Autodesk Fusion 360 part; units mm, degrees
sketch "Obturator" plane through (0, 0, 0) normal (1, 0, 0) x (0, 1, 0)
  circle A0 centre (0, 0) radius 80
  line L0 (85, 85) -> (-85, 85)
  line L1 (-85, 85) -> (-85, -85)
  line L2 (-85, -85) -> (85, -85)
  line L3 (85, -85) -> (85, 85)
  line L4 (85, 85) -> (-85, -85) construction
  line L5 (-85, 85) -> (85, -85) construction
  line L6 (-55, 55) -> (-30.5, 55)
  line L7 (-30.5, 55) -> (-30.5, 36)
  line L8 (-30.5, 36) -> (-55, 36)
  line L9 (-55, 36) -> (-55, 55)
  circle A1 centre (0, 0) radius 40
  line L10 (0, 0) -> (0, 80)
  line L11 (0, 0) -> (-80, 0)
  circle A2 centre (0, 0) radius 2.5
  dimension "d1" = 160
  dimension "d2" = 170
  dimension "d3" = 170
  dimension "d4" = 24.5
  dimension "d5" = 19
  dimension "d6" = 30
  dimension "d7" = 30
  dimension "d8" = 80
  dimension "d9" = 5
extrude "Extrude1" add sketch "Obturator" along normal blind 5 contours A0 A1 L10 L11 | A1 L10 L11 A2 | A1 L10 L11 A2 | L6 L7 L8 L9 picked at (-15.8593, 57.9262)
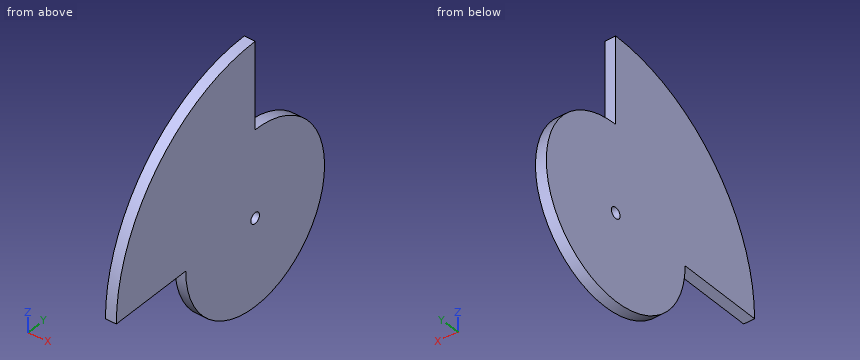
The model under review builds one solid part; all positions refer to its coordinate system, in mm. Round coordinates to 2 decimals unless told otherwise and drop trailing zeros. Write each loop counter-clockwise with the first axis right and the second up, starting at its lowest first coordinate (ties: lowest second). Pieces come first, ordered by that corner, then holes. Notation, with made-up numbers: (88, 43.5) -> (109, 43.5) arc R18 ccw to (109, 52.5) -> close; hole circle Ø9 at (72, -16). An arc over 180 degrees is marked (long way). Answer as a JSON object with one key per item and string values.
1. We need section B-B on z = -32.5. State the section outline as (x, y) points.
Results found:
{"outline": "(0, -23.32) -> (5, -23.32) -> (5, 23.32) -> (0, 23.32) -> close"}
2. We need section C-C on y = -12. State the section outline as (x, z) points.
Results found:
{"outline": "(0, -38.16) -> (5, -38.16) -> (5, 79.09) -> (0, 79.09) -> close"}
3. To check wall thickness, follow line 1 along Y through (x, z) = (4.3, 1); line 2 along Z through (x, y) = (0.45, -62.5); line 3 along Z through (x, y) = (2.3, -45.5). State the ranges of each line that lie inside material, in increasing order.
Results found:
{"line 1": "y = -79.99 to -2.29, 2.29 to 39.99", "line 2": "z = 0 to 49.94", "line 3": "z = 0 to 65.8"}
4. We need section A-A on x = 2.1. State the section outline as (y, z) points.
Results found:
{"outline": "(-80, 0) -> (-40, 0) arc R40 ccw (long way) to (0, 40) -> (0, 80) arc R80 ccw to start; hole circle Ø5 at (0, 0)"}
5. Clearance check with flat-ended pins moving along their axes: pin 1 (1.5 mm diameter, centred on x = 1, y = 18, fed in from +Z); pin 2 (1.5 mm diameter, centred on x = 1.5, z = 40.5, fed in from -Y); pin 3 (1.5 mm diameter, centred on x = 1.5, y = -60, fed in from -Z). State where each tip first meets the part, or that it passes through.
Results found:
{"pin 1": "stops at z = 36.09", "pin 2": "stops at y = -69.43", "pin 3": "stops at z = 0"}
